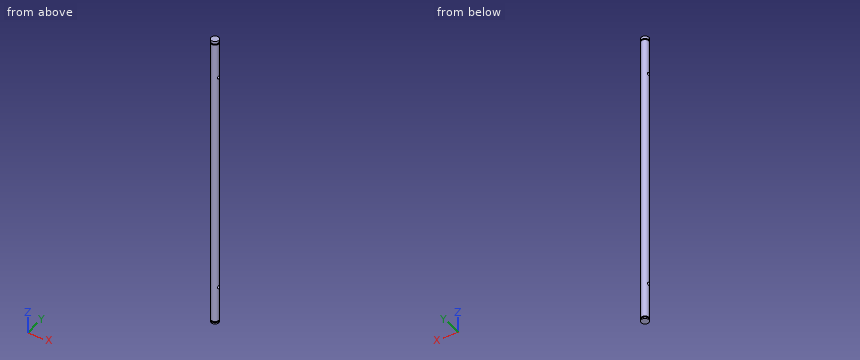
from build123d import *

# Parameters (mm, degrees)
SKETCH1_R           = 3
BOSS_EXTRUDE1_DEPTH = 233
SKETCH2_W           = 0.5
SKETCH2_H           = 1
CUT_EXTRUDE1_DEPTH  = 0.5
M3_TAPPED_HOLE1_D   = 2.5
SKETCH6_W           = 0.5
SKETCH6_H           = 1
BOSS_EXTRUDE2_DEPTH = 0.5


with BuildPart() as part:
    # Sketch1 → Boss-Extrude1 (new body)
    with BuildSketch(Plane.XY):
        Circle(SKETCH1_R)
    extrude(amount=BOSS_EXTRUDE1_DEPTH)

    # Sketch2 → Cut-Revolve1 (revolve, cut)
    with BuildSketch(Plane(origin=(0, 0, 0), x_dir=(1, 0, 0), z_dir=(0, 1, 0))):
        with Locations((2.75, -1.5)):
            Rectangle(SKETCH2_W, SKETCH2_H)
    revolve(axis=Axis((0, 0, 233), (0, 0, -1)), mode=Mode.SUBTRACT)

    # Sketch3 → Cut-Extrude1 (cut)
    with BuildSketch(Plane.XY.offset(233)):
        with BuildLine():
            Line((2.7, 1.307669683), (2.7, -1.307669683))
            ThreePointArc((2.7, -1.307669683), (3, 0), (2.7, 1.307669683))
        make_face()
    extrude(amount=-CUT_EXTRUDE1_DEPTH, mode=Mode.SUBTRACT)

    # M3 Tapped Hole1 (through all)
    with Locations(Plane(origin=(3.7, 0, 29.5), x_dir=(0, 0, 1), z_dir=(1, 0, 0))):
        with Locations((0, 0), (173, 0)):
            Hole(M3_TAPPED_HOLE1_D / 2)

    # Sketch6 → Cut-Revolve2 (revolve, cut)
    with BuildSketch(Plane(origin=(0, 0, 0), x_dir=(1, 0, 0), z_dir=(0, 1, 0))):
        with Locations((2.75, -230.5)):
            Rectangle(SKETCH6_W, SKETCH6_H)
    revolve(axis=Axis((0, 0, 233), (0, 0, -1)), mode=Mode.SUBTRACT)

    # Sketch7 → Boss-Extrude2 (add)
    with BuildSketch(Plane.XY.offset(232.5)):
        with BuildLine():
            Line((2.7, 1.307669683), (2.7, -1.307669683))
            ThreePointArc((2.7, -1.307669683), (3, 0), (2.7, 1.307669683))
        make_face()
    extrude(amount=BOSS_EXTRUDE2_DEPTH)


solid = part.part
Geometry check sheet. Reference: the model listing, model coordinates, mm. Round coordinates to 2 decimals unless told otherwise and drop trailing zeros. Order: outer loops, then holes, each group sorted by start corner. A loop starts at its lowest first (then second) coordinate and runs counter-clockwise, first axis right, second up. Notation, with made-up numbers: M 66.25,2.5 L 88.25,2.5 A11 ccw 88.25,14.5 Z; hole C 85,25.5 d1. An arc over 180 degrees is marked long. Answer in a Markdown table with one row per item. Add a question column.
Item 1: Sectioned sample at A-A, the plane y = 0. Enter the section's corners in (x, z).
Item 2: Depth check by flat-ended pin: pin 1 Ø1 at (y, z) = (1.5, 113) entering from +X; pin 2 Ø1.5 at (y, z) = (0, 29.5) entering from -X. Enter the tip coordinate at first touch or a pass-through.
Item 3: Material ranges on L1, parallel to Z at x = -1, y = -1; L2, parallel to Z at x = -2, y = 0.5; L3, parallel to Y at x = 0, z = 202.5, recorded low to high. Write a range as [from, to].
Item 4: Sectioned sample at C-C, the plane z = 18. Enter the section's corners in (x, y), plus the area to 3 significant figures.
Item 5: Sectioned sample at B-B, the plane x = 1.5. Enter the section's corners in (y, z), plus the area to 3 significant figures.
Filled in:
| question | item | result |
|---|---|---|
| 1 | outline | M -3,0 L 3,0 L 3,1 L 2.5,1 L 2.5,2 L 3,2 L 3,28.25 L -3,28.25 L -3,2 L -2.5,2 L -2.5,1 L -3,1 Z; M -3,30.75 L 3,30.75 L 3,201.25 L -3,201.25 Z; M -3,203.75 L 3,203.75 L 3,230 L 2.5,230 L 2.5,231 L 3,231 L 3,233 L -3,233 L -3,231 L -2.5,231 L -2.5,230 L -3,230 Z |
| 2 | pin 1 | stops at x = 2.83 |
| 2 | pin 2 | passes through |
| 3 | L1 | z = [0, 28.75], [30.25, 201.75], [203.25, 233] |
| 3 | L2 | z = [0, 28.35], [30.65, 201.35], [203.65, 233] |
| 3 | L3 | y = [-3, -1.25], [1.25, 3] |
| 4 | outline | C 0,0 d6 |
| 4 | area | 28.3 mm² |
| 5 | outline | M -2.6,0 L 2.6,0 L 2.6,1 L 2,1 L 2,2 L 2.6,2 L 2.6,230 L 2,230 L 2,231 L 2.6,231 L 2.6,233 L -2.6,233 L -2.6,231 L -2,231 L -2,230 L -2.6,230 L -2.6,2 L -2,2 L -2,1 L -2.6,1 Z; hole C 0,29.5 d2.5; hole C 0,202.5 d2.5 |
| 5 | area | 1,200 mm² |
